Verification items for this drawing (mm, ordinates from the low corner). A direction names the side the tool comes from. Give positions to 0.01 mm unless a question says otherwise; leave off trailing zeros. Loops run counter-clockwise (first coordinate to the right, second up) from the corner with the lowest first, then second, coordinate; pieces in that order, holes last. Notation, with made-up numbers: M 29,-18 L 51,-18 A34 ccw 51,17 Z; hole C 83,1.5 d8. An arc over 180 degrees is marked long. Use one line per item in the form item = value.
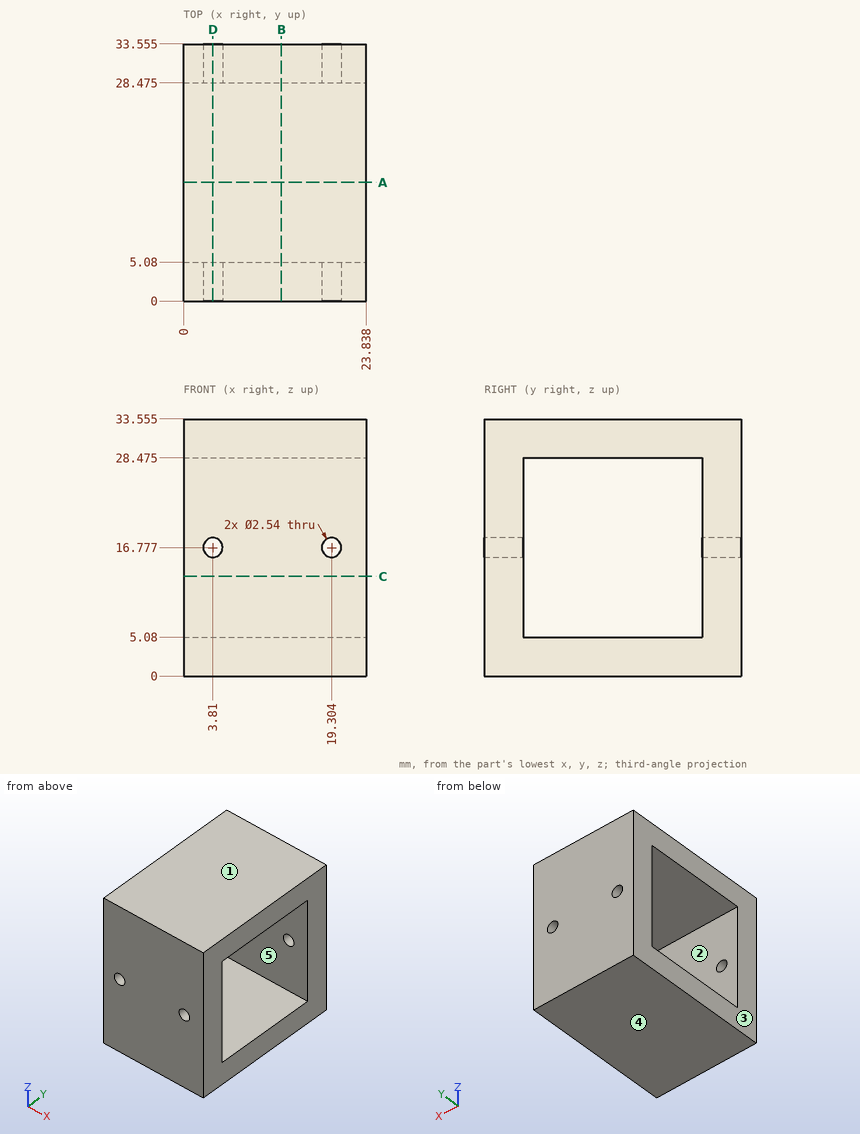
1) Release check for a two-part mould opening along Z. For the marked faces 3, 4 and 5 record: pulls with the +Z half, pulls with the -Z half, needs draft (parallel to the pull), parting line crosses it, or undercut.
Evaluation:
face_3 = needs draft
face_4 = pulls with the -Z half
face_5 = undercut
2) Section check D-D (x = 3.81). Record the cut outline in (y, z) (1 decimal), then the cut area to 3 significant figures.
Evaluation:
outline = M 0,0 L 33.6,0 L 33.6,15.5 L 28.5,15.5 L 28.5,5.1 L 5.1,5.1 L 5.1,15.5 L 0,15.5 Z; M 0,18 L 5.1,18 L 5.1,28.5 L 28.5,28.5 L 28.5,18 L 33.6,18 L 33.6,33.6 L 0,33.6 Z
area = 553 mm^2
3) Section check B-B (x = 12.75). Record the cut outline in (y, z) (1 decimal).
Evaluation:
outline = M 0,0 L 33.6,0 L 33.6,33.6 L 0,33.6 Z; hole M 5.1,5.1 L 28.5,5.1 L 28.5,28.5 L 5.1,28.5 Z
4) Depth check by flat-ended pin: pin 1 Ø1.5 at (x, z) = (3.81, 16.78) entering from -Y; pin 2 Ø6 at (y, z) = (26, 21.5) entering from +X. Enter the tip coordinate at first touch or a pass-through.
Evaluation:
pin_1 = through
pin_2 = 23.84
5) Section check A-A (y = 15.5). Record the cut outline in (x, z) (1 decimal), then the cut area to 3 significant figures.
Evaluation:
outline = M 0,0 L 23.8,0 L 23.8,5.1 L 0,5.1 Z; M 0,28.5 L 23.8,28.5 L 23.8,33.6 L 0,33.6 Z
area = 242 mm^2
6) Scan lines: line 1 (Y direction, x = 3.75, z = 21) (1 decimal); line 2 (X direction, y = 3.5, z = 16) (1 decimal). Record each from-to range of solid material in increasing order.
Evaluation:
line_1 = 0 to 5.1, 28.5 to 33.6
line_2 = 0 to 2.8, 4.8 to 18.3, 20.3 to 23.8
7) Set-up check for the marked faces 1 and 2: record each of +Z, -Z, +X, -X, +Y, -Y from which the full face is reachable in a straight line by a thin tool's end or side.
Evaluation:
face_1 = +Z, +X, -X, +Y, -Y
face_2 = +X, -X
